Source: CAD feature listing. Evaluate the final solid. Frame: model axes, mm. A direction names the side the tool comes from. Round coordinates to 2 decimals unless told otherwise and drop trailing zeros. Write each loop counter-clockwise with the first axis right and the second up, starting at its lowest first coordinate (ties: lowest second). Pieces come first, ordered by that corner, then holes. Notation, with made-up numbers: M 55.5,-9 L 71.5,-9 A4 cw 71.5,-2 Z; hole C 72,-3 d11. An arc over 180 degrees is marked long. Answer in a Markdown table with one row per item.
from build123d import *

# Parameters (mm, degrees)
F3_D = 12.7


with BuildPart() as f1:
    # F0 (on Front) → F1 (revolve)
    with BuildSketch(Plane.XZ):
        Polygon((4.7498, 0), (0, 0), (0, -31.75), (0.762, -31.75), (0.762, -44.45), (0, -44.45), (0, -76.2), (4.7498, -76.2), (4.7498, -44.45), (3.9878, -44.45), (3.9878, -31.75), (4.7498, -31.75), align=None)
    revolve(axis=Axis((20.701, 0, -38.1), (0, 0, -1)))

    # F3 (through all)
    with Locations(Plane(origin=(0, 0, 0), x_dir=(0, 1, 0), z_dir=(-1, 0, 0))):
        with Locations((0, 38.1)):
            Hole(F3_D / 2)


solid = f1.part
Q1. Contact query for flat-ended pins moving along their axis: pin 1 Ø4 at (x, z) = (8.5, -55.5) entering from +Y; pin 2 Ø3 at (x, z) = (25.5, -65) entering from +Y; pin 3 Ø10 at (x, y) = (23, 5.5) entering from +Z; pin 4 Ø8 at (y, z) = (-13, -37.5) entering from +X. Output: stop coordinate, or through.
Solutions:
| item | result |
|---|---|
| pin 1 | stops at y = 18.01 |
| pin 2 | stops at y = 20.44 |
| pin 3 | passes through |
| pin 4 | stops at x = 38.49 |
Q2. Section D-D (y = -2.5). State how many separate pieces and enclosed holes the cut face has, and give its area (3 significant figures).
Solutions:
| item | result |
|---|---|
| separate pieces | 4 |
| enclosed holes | 0 |
| area | 616 mm2 |
Q3. Section A-A (y = -13). Return loops of the section in (x, z).
Solutions:
| item | result |
|---|---|
| outline | M 4.59,-76.2 L 11.46,-76.2 L 11.46,-44.45 L 10.2,-44.45 L 10.2,-31.75 L 11.46,-31.75 L 11.46,0 L 4.59,0 L 4.59,-31.75 L 5.58,-31.75 L 5.58,-44.45 L 4.59,-44.45 Z; M 29.94,-76.2 L 36.81,-76.2 L 36.81,-44.45 L 35.82,-44.45 L 35.82,-31.75 L 36.81,-31.75 L 36.81,0 L 29.94,0 L 29.94,-31.75 L 31.2,-31.75 L 31.2,-44.45 L 29.94,-44.45 Z |
Q4. Access query for faces 4 (the cylindrical face through (21.139, -19.934, -38.189)), 5 (the cylindrical face through (32.46, 10.78, -15.65)), 6 (the cylindrical face through (20.33, 16.71, -38.01)). Directions: +Z, -Z, +X, -X, +Y, -Y. A direction counts if a zero-diameter tool reaches every point of the face in a straight line with its end or side. Return the directions, or none.
Solutions:
| item | result |
|---|---|
| face 4 | -Y |
| face 5 | +Z, -Z |
| face 6 | none |
Q5. Section B-B (z = -33). Return loops of the section in (x, y).
Solutions:
| item | result |
|---|---|
| outline | M 1.12,-3.78 A19.94 ccw 40.28,-3.78 L 36.98,-3.78 A16.71 cw 4.42,-3.78 Z; M 1.12,3.78 L 4.42,3.78 A16.71 cw 36.98,3.78 L 40.28,3.78 A19.94 ccw Z |
Q6. Section C-C (x = 15). Return loops of the section in (y, z).
Solutions:
| item | result |
|---|---|
| outline | M -19.9,-76.2 L -14.9,-76.2 L -14.9,-44.45 L -15.71,-44.45 L -15.71,-31.75 L -14.9,-31.75 L -14.9,0 L -19.9,0 L -19.9,-31.75 L -19.11,-31.75 L -19.11,-44.45 L -19.9,-44.45 Z; M 14.9,-76.2 L 19.9,-76.2 L 19.9,-44.45 L 19.11,-44.45 L 19.11,-31.75 L 19.9,-31.75 L 19.9,0 L 14.9,0 L 14.9,-31.75 L 15.71,-31.75 L 15.71,-44.45 L 14.9,-44.45 Z |
Q7. Material intervals for probe 1 along Z at (x, y) = (2, 8); probe 2 along Y at (x, z) = (12, -65); probe 3 along Y at (x, z) = (19, -68.5), sorted ascending.
Solutions:
| item | result |
|---|---|
| probe 1 | z = -76.2 to -44.45, -31.75 to 0 |
| probe 2 | y = -18.78 to -13.37, 13.37 to 18.78 |
| probe 3 | y = -20.63 to -15.86, 15.86 to 20.63 |
Q8. Pull-direction query (Y, two-part tool) for faces 1 (the flat face through (9.9, 17, -44.45)), 2 (the cylindrical face through (37.129, -12.596, -60.547)), 3 (the cylindrical face through (21.07, -16.71, -38.01)); classes: pulls with the +Y half, pulls with the -Y half, needs draft (parallel to the pull), parting line crosses it, or undercut.
Solutions:
| item | result |
|---|---|
| face 1 | needs draft |
| face 2 | parting line crosses it |
| face 3 | undercut |
